from build123d import *

# Parameters (mm, degrees)
SZKIC1_W                        = 10
SZKIC1_H                        = 15
DODANIE_WYCI_GNI_CIE1_DEPTH     = 50
SZKIC2_W                        = 10
SZKIC2_H                        = 15
DODANIE_WYCI_GNI_CIE2_DEPTH     = 47
SZKIC3_R                        = 1.6
WYTNIJ_WYCI_GNI_CIE1_DEPTH      = 54.217463596
SZKIC4_R                        = 3
WYTNIJ_WYCI_GNI_CIE2_DEPTH      = 3
SZKIC5_R                        = 1.15
WYTNIJ_WYCI_GNI_CIE3_DEPTH      = 10
WYTNIJ_WYCI_GNI_CIE4_DEPTH      = 51.91835936
WYTNIJ_WYCI_GNI_CIE4_DEPTH_BACK = 51.91835936
SZKIC7_R                        = 3


with BuildPart() as part:
    # Szkic1 → Dodanie-wyciągnięcie1 (new body)
    with BuildSketch(Plane.XY):
        with Locations((5.348837209, 0.726744186)):
            Rectangle(SZKIC1_W, SZKIC1_H)
    extrude(amount=DODANIE_WYCI_GNI_CIE1_DEPTH)

    # Szkic2 → Dodanie-wyciągnięcie2 (add)
    with BuildSketch(Plane(origin=(0, 0, 0), x_dir=(-1, 0, 0), z_dir=(0, 0, -1))):
        with Locations((-5.348837209, 0.726744186)):
            Rectangle(SZKIC2_W, SZKIC2_H)
    extrude(amount=DODANIE_WYCI_GNI_CIE2_DEPTH)

    # Szkic3 → Wytnij-wyciągnięcie1 (cut, through all)
    with BuildSketch(Plane(origin=(0, 8.226744186, 0), x_dir=(1, 0, 0), z_dir=(0, 1, 0))):
        with Locations(Location((5.348837209, 30.75, 0), (0, 0, 270))):
            Circle(SZKIC3_R)
        with Locations(Location((5.348837209, -33.75, 0), (0, 0, 270))):
            Circle(SZKIC3_R)
    extrude(amount=-WYTNIJ_WYCI_GNI_CIE1_DEPTH, mode=Mode.SUBTRACT)

    # Szkic4 → Wytnij-wyciągnięcie2 (cut)
    with BuildSketch(Plane.XZ.offset(6.773255814)):
        with Locations(Location((5.348837209, -30.75, 0), (0, 0, 270))):
            Circle(SZKIC4_R)
        with Locations(Location((5.348837209, 33.75, 0), (0, 0, 270))):
            Circle(SZKIC4_R)
    extrude(amount=-WYTNIJ_WYCI_GNI_CIE2_DEPTH, mode=Mode.SUBTRACT)

    # Szkic5 → Wytnij-wyciągnięcie3 (cut)
    with BuildSketch(Plane.XY.offset(50)):
        with Locations((5.348837209, 0.726744186)):
            Circle(SZKIC5_R)
    extrude(amount=-WYTNIJ_WYCI_GNI_CIE3_DEPTH, mode=Mode.SUBTRACT)

    # Szkic7 → Wytnij-wyciągnięcie4 (cut, two sides: drawn at the far end of the back side and taken through both)
    with BuildSketch(Plane.ZY.offset(-5.348837209).offset(-WYTNIJ_WYCI_GNI_CIE4_DEPTH_BACK)):
        with Locations((27.792952472, 0.629031613)):
            Circle(SZKIC7_R)
        with Locations((14.792952472, 0.629031613)):
            Circle(SZKIC7_R)
        with Locations((1.792952472, 0.629031613)):
            Circle(SZKIC7_R)
        with Locations((-11.207047528, 0.629031613)):
            Circle(SZKIC7_R)
        with Locations((-24.207047528, 0.629031613)):
            Circle(SZKIC7_R)
        with Locations((-37.207047528, 0.629031613)):
            Circle(SZKIC7_R)
    extrude(amount=WYTNIJ_WYCI_GNI_CIE4_DEPTH + WYTNIJ_WYCI_GNI_CIE4_DEPTH_BACK, mode=Mode.SUBTRACT)


solid = part.part
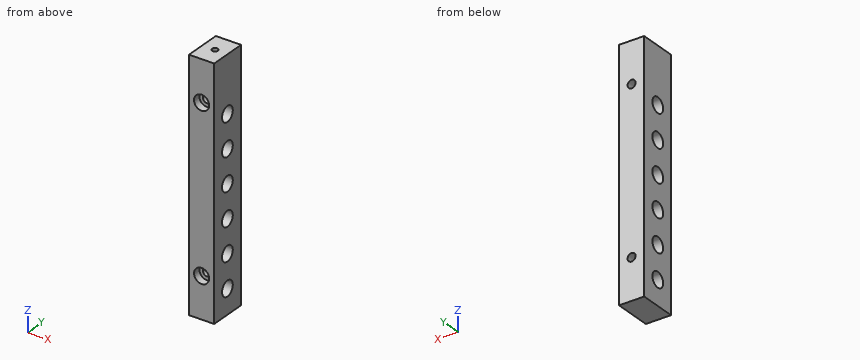
Could you check a few things on this model? Use its own coordinates, in mm. Coordinates: 2 decimals unless noted, no trailing zeros. Loops run counter-clockwise (first coordinate to the right, second up) from the corner with the lowest first, then second, coordinate; pieces in that order, holes last. Notation, with made-up numbers: (63.5, 50.5) -> (116.5, 50.5) arc R9 ccw to (116.5, 64.5) -> close; hole circle Ø5 at (-13, -25.5). An arc over 180 degrees is marked (long way). Answer in a Markdown table with one row per item.
(1) Imagine slicing it at A-A (z = -30.75). List the corners of the cut face in (x, y) for me.
Results found:
| item | result |
|---|---|
| outline | (0.35, -6.77) -> (2.35, -6.77) -> (2.35, -3.77) -> (3.75, -3.77) -> (3.75, 8.23) -> (0.35, 8.23) -> close; (6.95, -3.77) -> (8.35, -3.77) -> (8.35, -6.77) -> (10.35, -6.77) -> (10.35, 8.23) -> (6.95, 8.23) -> close |
(2) Imagine slicing it at C-C (z = 1.5). List the corners of the cut face in (x, y) for me.
Results found:
| item | result |
|---|---|
| outline | (0.35, -6.77) -> (10.35, -6.77) -> (10.35, -2.36) -> (0.35, -2.36) -> close; (0.35, 3.61) -> (10.35, 3.61) -> (10.35, 8.23) -> (0.35, 8.23) -> close |
(3) Imagine slicing it at B-B (y = 5). List the corners of the cut face in (x, z) for me.
Results found:
| item | result |
|---|---|
| outline | (0.35, -47) -> (10.35, -47) -> (10.35, 50) -> (0.35, 50) -> close; hole circle Ø3.2 at (5.35, -30.75); hole circle Ø3.2 at (5.35, 33.75) |
(4) Imagine slicing it at D-D (z = 13). List the corners of the cut face in (x, y) for me, plus the area to 3 significant figures.
Results found:
| item | result |
|---|---|
| outline | (0.35, -6.77) -> (10.35, -6.77) -> (10.35, -1.78) -> (0.35, -1.78) -> close; (0.35, 3.03) -> (10.35, 3.03) -> (10.35, 8.23) -> (0.35, 8.23) -> close |
| area | 102 mm^2 |
(5) If I drill on probe 1 along Z at (x, y) = (5.25, 5); probe 2 along X at (y, z) = (-0.5, -30.75); probe 3 along X at (y, z) = (4.75, -30.5), over which ranges is the centre line in solid material (lowest first)?
Results found:
| item | result |
|---|---|
| probe 1 | z = -47 to -32.35, -29.15 to 32.15, 35.35 to 50 |
| probe 2 | x = 0.35 to 3.75, 6.95 to 10.35 |
| probe 3 | x = 0.35 to 3.77, 6.93 to 10.35 |
(6) Will this pin go through, and if not, where does the flat tip stop? pin 1 Ø3 at (x, z) = (4.5, 34) entering from -Y.
Results found:
| item | result |
|---|---|
| pin 1 | stops at y = -3.77 |
